The listing builds one solid part. Answer for the finished solid, in the listing's coordinates (mm). A direction names the side the tool comes from. Coordinates: 2 decimals unless noted, no trailing zeros. Loops run counter-clockwise (first coordinate to the right, second up) from the corner with the lowest first, then second, coordinate; pieces in that order, holes last. Notation, with made-up numbers: M 84,22 L 91,22 A22 ccw 91,34 Z; hole C -32.75,-17 d5. An arc over 180 degrees is marked long. Answer in a Markdown table with one row per item. Add a question column.
from build123d import *

# Parameters (mm, degrees)
CROQUIS1_W                   = 2.25
CROQUIS1_H                   = 46
SALIENTE_EXTRUIR1_DEPTH      = 7
SALIENTE_EXTRUIR1_DEPTH_BACK = 7
CROQUIS2_R                   = 2.5
REDONDEO3_R                  = 0.5


with BuildPart() as part:
    # Croquis1 → Revoluci_n1 (revolve)
    with BuildSketch(Plane.XY, mode=Mode.PRIVATE) as revoluci_n1_sk:
        with Locations((1.125, 23)):
            Rectangle(CROQUIS1_W, CROQUIS1_H)
    revolve(revoluci_n1_sk.sketch.rotate(Axis((0, 0, 0), (0, 1, 0)), 90), axis=Axis((0, 0, 0), (0, 1, 0)))

    # Croquis2 → Saliente-Extruir1 (add, two sides: drawn at the far end of the back side and taken through both)
    with BuildSketch(Plane(origin=(0, 0, 0), x_dir=(0, 0, -1), z_dir=(1, 0, 0)).offset(-SALIENTE_EXTRUIR1_DEPTH_BACK)):
        with Locations((0, 46)):
            Circle(CROQUIS2_R)
    extrude(amount=SALIENTE_EXTRUIR1_DEPTH + SALIENTE_EXTRUIR1_DEPTH_BACK)

    # Redondeo3
    redondeo3_edges = [part.edges().sort_by_distance(p)[0] for p in [
        (2.25, 43.5, 0),
    ]]
    fillet(redondeo3_edges, radius=REDONDEO3_R)


solid = part.part
(1) For faces 1 (the face through (-0.1, 48.48, 0.33)), 2 (the face through (7, 46, 0)), 3 (the face through (-0.676, 22.714, -2.146)), determine the directions among +Z, -Z, +X, -X, +Y, -Y from which every point of the face is accessible in a straight line to the end or side of a thin tool.
(2) Each of these flat-tipped pins is pushed along its axis until it touches: pin 1 (8 mm diameter, centred on x = -2.5, y = 13, fed in from -Z); pin 2 (1 mm diameter, centred on x = 1, z = -1, fed in from +Y); pin 3 (2 mm diameter, centred on y = 12.5, z = 1, fed in from -X). Where does it stop, or does it pass through?
(3) A cutting plane is placed at B-B (y = 23). Give the vertices of the cut face in (x, z).
(4) Straight lines are drawn through the part: line 1 (X direction, y = 25, z = -0.2); line 2 (Y direction, x = 2, z = -0.1); line 3 (Y direction, x = 0, z = -0.7). For each, find the intervals that lie inside material, in ascending order.
(5) A cutting plane is placed at A-A (x = 5.5). Give the vertices of the cut face in (y, z), plus the area to 3 significant figures.
Solved:
| question | item | result |
|---|---|---|
| 1 | face 1 | none |
| 1 | face 2 | +Z, -Z, +X, +Y, -Y |
| 1 | face 3 | -Y |
| 2 | pin 1 | stops at z = -2.25 |
| 2 | pin 2 | stops at y = 48.45 |
| 2 | pin 3 | stops at x = -2.25 |
| 3 | outline | C 0,0 d4.5 |
| 4 | line 1 | x = -2.24 to 2.24 |
| 4 | line 2 | y = 0 to 48.5 |
| 4 | line 3 | y = 0 to 48.4 |
| 5 | outline | C 46,0 d5 |
| 5 | area | 19.6 mm² |
